Could you check a few things on this model? Use its own coordinates, in mm. Round coordinates to 2 decimals unless told otherwise and drop trailing zeros. Loops run counter-clockwise (first coordinate to the right, second up) from the corner with the lowest first, then second, coordinate; pieces in that order, holes last. Notation, with made-up numbers: (26, -10) -> (68, -10) arc R24 ccw to (68, 0) -> close; hole circle Ø8 at (37, -30.75). An arc over 180 degrees is marked (long way). Put each result on its own line as item: value. Start each with the question number.
1. Imagine slicing it at C-C, the plane x = -15.5. Please give me the cut outline in (y, z).
2. Imagine slicing it at D-D, the plane y = 1.25. Please give me the cut outline in (x, z).
3. I need wall thicknesses on line 1 (Z direction, x = 3, y = 7); line 2 (Y direction, x = -12, z = -9); line 3 (X direction, y = 13, z = -17). Which ranges of each line are inside material? Lowest first, please. Write a range as [from, to].
4. Imagine slicing it at B-B, the plane x = -0.5. Please give me the cut outline in (y, z).
5. Imagine slicing it at A-A, the plane z = 17. Please give me the cut outline in (x, y).
6. I'm going to push a flat-ended pin straight in: P1, Ø1.5, axis at y = 7.5, z = 8, coming from the -X side. Where does the tip first touch, or does it pass through?
```python
from build123d import *

# Parameters (mm, degrees)
SKETCH_1_W          = 61
SKETCH_1_H          = 42
EXTRUDE_1_DEPTH     = 17
SKETCH_2_R          = 1.75
CUT_EXTRUDE_1_DEPTH = 17
SKETCH_3_R          = 2.5
CUT_EXTRUDE_2_DEPTH = 45


with BuildPart() as part:
    # 草图1 → 凸台-拉伸1 (new body)
    with BuildSketch(Plane(origin=(0, 0, 0), x_dir=(1, 0, 0), z_dir=(0, 1, 0))):
        Rectangle(SKETCH_1_W, SKETCH_1_H)
    extrude(amount=EXTRUDE_1_DEPTH)

    # 草图2 → 切除-拉伸1 (cut)
    with BuildSketch(Plane(origin=(0, 17, 0), x_dir=(1, 0, 0), z_dir=(0, 1, 0))):
        with Locations(Location((-0.5, 17, 0), (0, 0, 270))):
            Circle(SKETCH_2_R)
        with Locations(Location((-0.5, -17, 0), (0, 0, 270))):
            Circle(SKETCH_2_R)
        with Locations(Location((-15.5, 0, 0), (0, 0, 270))):
            Circle(SKETCH_2_R)
        with Locations(Location((9.5, 0, 0), (0, 0, 270))):
            Circle(SKETCH_2_R)
    extrude(amount=-CUT_EXTRUDE_1_DEPTH, mode=Mode.SUBTRACT)

    # 草图3 → 切除-拉伸2 (cut)
    with BuildSketch(Plane.ZY.offset(30.5)):
        with Locations((-9, 8.5)):
            Circle(SKETCH_3_R)
        with Locations((9, 8.5)):
            Circle(SKETCH_3_R)
    extrude(amount=-CUT_EXTRUDE_2_DEPTH, mode=Mode.SUBTRACT)


solid = part.part
```
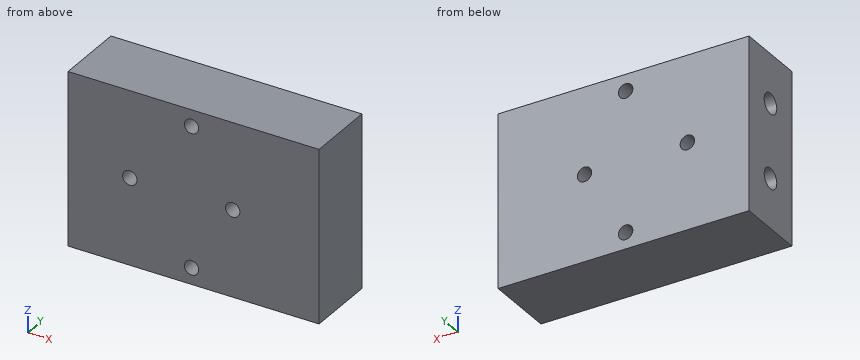
Entries:
1. outline: (0, -21) -> (17, -21) -> (17, -1.75) -> (0, -1.75) -> close; (0, 1.75) -> (17, 1.75) -> (17, 21) -> (0, 21) -> close; hole circle Ø5 at (8.5, -9); hole circle Ø5 at (8.5, 9)
2. outline: (-30.5, -21) -> (30.5, -21) -> (30.5, 21) -> (-30.5, 21) -> close; hole circle Ø3.5 at (-15.5, 0); hole circle Ø3.5 at (-0.5, -17); hole circle Ø3.5 at (-0.5, 17); hole circle Ø3.5 at (9.5, 0)
3. line 1: [-21, -11], [-7, 7], [11, 21]
3. line 2: [0, 6], [11, 17]
3. line 3: [-30.5, -2.25], [1.25, 30.5]
4. outline: (0, -21) -> (17, -21) -> (17, -18.75) -> (0, -18.75) -> close; (0, -15.25) -> (17, -15.25) -> (17, 15.25) -> (0, 15.25) -> close; (0, 18.75) -> (17, 18.75) -> (17, 21) -> (0, 21) -> close; hole circle Ø5 at (8.5, -9); hole circle Ø5 at (8.5, 9)
5. outline: (-30.5, 0) -> (-2.25, 0) -> (-2.25, 17) -> (-30.5, 17) -> close; (1.25, 0) -> (30.5, 0) -> (30.5, 17) -> (1.25, 17) -> close
6. P1: x = 14.5
